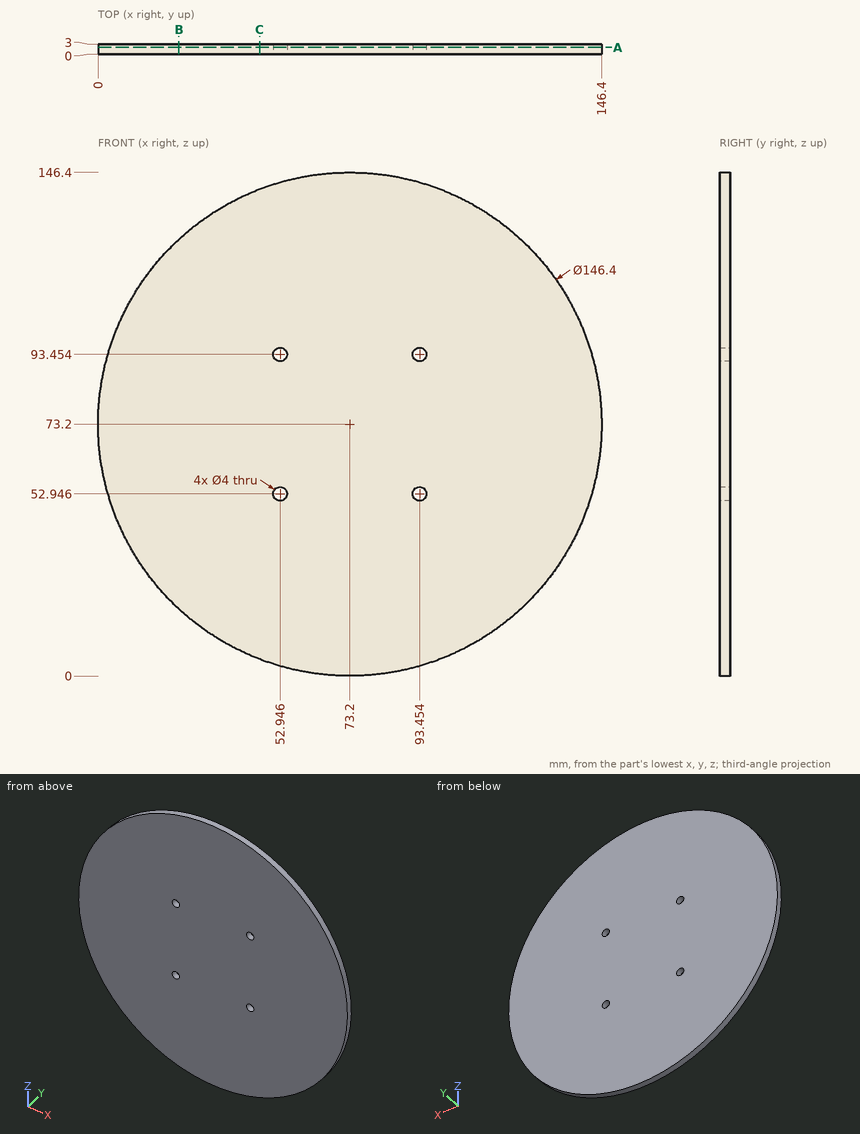
Drawing for the job (mm, zero at the part's lowest x, y, z). Round coordinates to 2 decimals unless told otherwise and drop trailing zeros. Write each loop counter-clockwise with the first axis right and the second up, starting at its lowest first coordinate (ties: lowest second). Pieces come first, ordered by that corner, then holes. Notation, with made-up numbers: (70.5, 52) - (118.5, 52) arc R34 ccw to (118.5, 88) - close; hole circle Ø1 at (44, 55.25). An arc over 180 degrees is marked (long way). Return JSON: item names as keys, results as strings. Group by question number.
Item 1: Band-saw the part on B-B on x = 23.5. List the corners of the cut face in (y, z).
Item 2: Band-saw the part on A-A on y = 2.05. List the corners of the cut face in (x, z), plus the area to 3 significant figures.
Item 3: Band-saw the part on C-C on x = 47. List the corners of the cut face in (y, z), plus the area to 3 significant figures.
Item 4: Probe probe 1 along X at (y, z) = (1, 55.5); probe 2 along X at (y, z) = (1.75, 64.5); probe 3 along Z at (x, y) = (131, 0.65) (1 decimal). List the from-to ranges inside material, lowest first.
Item 5: Flat gauge pins, fed straight in: pin 1 Ø1.5 at (y, z) = (1.5, 81) entering from -X; pin 2 Ø1.5 at (x, y) = (78.5, 1) entering from -Z; pin 3 Ø1.5 at (x, y) = (111, 2) entering from +Z. Where does each tip first touch, or does it go through?
Resolved:
{
 "1": {"outline": "(0, 19.46) - (3, 19.46) - (3, 126.94) - (0, 126.94) - close"},
 "2": {"outline": "circle Ø146.4 at (73.2, 73.2); hole circle Ø4 at (52.95, 52.95); hole circle Ø4 at (52.95, 93.45); hole circle Ø4 at (93.45, 52.95); hole circle Ø4 at (93.45, 93.45)", "area": "16,800 mm²"},
 "3": {"outline": "(0, 4.85) - (3, 4.85) - (3, 141.55) - (0, 141.55) - close", "area": "410 mm²"},
 "4": {"probe 1": "x = 2.17 to 144.23", "probe 2": "x = 0.52 to 145.88", "probe 3": "z = 28.3 to 118.1"},
 "5": {"pin 1": "stops at x = 0.34", "pin 2": "stops at z = 0.14", "pin 3": "stops at z = 136.33"}
}
